Here's how the part is built. I have some questions about the finished solid (model axes, mm). Face numbers are marked on the shaded views. A direction names the side the tool comes from. Coordinates: 2 decimals unless noted, no trailing zeros. Loops run counter-clockwise (first coordinate to the right, second up) from the corner with the lowest first, then second, coordinate; pieces in that order, holes last. Notation, with made-up numbers: (29.25, 20.5) - (72.25, 20.5) arc R10 cw to (72.25, 24.5) - close; hole circle Ø7 at (18, 17). An arc over 180 degrees is marked (long way). Use a Markdown table: item, result.
```python
from build123d import *

# Parameters (mm, degrees)
SKETCH_W        = 59
SKETCH_H        = 60
PAD_DEPTH       = 11
SKETCH001_R     = 7.6
POCKET_DEPTH    = 60.001
SKETCH002_R     = 1.75
POCKET001_DEPTH = 11.001
POCKET002_DEPTH = 9
SKETCH004_R     = 2.25
POCKET003_DEPTH = 11.001
SKETCH008_R     = 4.1
POCKET005_DEPTH = 20
SKETCH010_W     = 20
SKETCH010_H     = 25
POCKET006_DEPTH = 5
SKETCH011_R     = 2.9
POCKET007_DEPTH = 3.5
CHAMFER_SIZE    = 3


with BuildPart() as part:
    # Sketch → Pad (new body)
    with BuildSketch(Plane.XY):
        with Locations((19.5, 0)):
            Rectangle(SKETCH_W, SKETCH_H)
    extrude(amount=PAD_DEPTH)

    # Sketch001 → Pocket (cut, through all)
    with BuildSketch(Plane.XZ.offset(30)):
        with Locations((0, 11)):
            Circle(SKETCH001_R)
    extrude(amount=-POCKET_DEPTH, mode=Mode.SUBTRACT)

    # Sketch002 → Pocket001 (cut, through all)
    with BuildSketch(Plane.XY.offset(11)):
        with Locations((-6, 27)):
            Circle(SKETCH002_R)
        with Locations((40, 27)):
            Circle(SKETCH002_R)
        with Locations((-6, -27)):
            Circle(SKETCH002_R)
        with Locations((40, -27)):
            Circle(SKETCH002_R)
        with Locations((6, 27)):
            Circle(SKETCH002_R)
        with Locations((6, -27)):
            Circle(SKETCH002_R)
        with Locations((6, 0)):
            Circle(SKETCH002_R)
        with Locations((-6, 0)):
            Circle(SKETCH002_R)
        with Locations((40, -13)):
            Circle(SKETCH002_R)
        with Locations((40, 13)):
            Circle(SKETCH002_R)
    extrude(amount=-POCKET001_DEPTH, mode=Mode.SUBTRACT)

    # Sketch003 → Pocket002 (cut)
    with BuildSketch(Plane.XY.offset(11)):
        with BuildLine():
            Line((10, 35), (10, -35))
            Line((10, -35), (32, -35))
            Line((32, -35), (32, -17.246794))
            ThreePointArc((32, -17.246794), (35.044647, -14.065445), (36.736695, -10))
            Line((36.736695, -10), (56.736695, -10))
            Line((56.736695, -10), (56.736695, 10))
            Line((56.736695, 10), (36.736695, 10))
            ThreePointArc((36.736695, 10), (35.044647, 14.065445), (32, 17.246794))
            Line((32, 17.246794), (32, 35))
            Line((32, 35), (10, 35))
        make_face()
    extrude(amount=-POCKET002_DEPTH, mode=Mode.SUBTRACT)

    # Sketch004 → Pocket003 (cut, through all)
    with BuildSketch(Plane(origin=(0, 0, 0), x_dir=(1, 0, 0), z_dir=(0, 0, -1))):
        with Locations((25, 7.5)):
            Circle(SKETCH004_R)
        with Locations((25, -7.5)):
            Circle(SKETCH004_R)
    extrude(amount=-POCKET003_DEPTH, mode=Mode.SUBTRACT)

    # Sketch008 → Pocket005 (cut)
    with BuildSketch(Plane.YZ.offset(49)):
        with Locations((-20, 11)):
            Circle(SKETCH008_R)
        with Locations((20, 11)):
            Circle(SKETCH008_R)
    extrude(amount=-POCKET005_DEPTH, mode=Mode.SUBTRACT)

    # Sketch010 → Pocket006 (cut)
    with BuildSketch(Plane.YZ.offset(49)):
        with Locations((0, 5.473744)):
            Rectangle(SKETCH010_W, SKETCH010_H)
    extrude(amount=-POCKET006_DEPTH, mode=Mode.SUBTRACT)

    # Sketch011 → Pocket007 (cut)
    with BuildSketch(Plane(origin=(0, 0, 0), x_dir=(1, 0, 0), z_dir=(0, 0, -1))):
        with Locations((6, 27)):
            Circle(SKETCH011_R)
        with Locations((40, -13)):
            Circle(SKETCH011_R)
        with Locations((-6, -27)):
            Circle(SKETCH011_R)
        with Locations((6, -27)):
            Circle(SKETCH011_R)
        with Locations((40, 27)):
            Circle(SKETCH011_R)
        with Locations((40, 13)):
            Circle(SKETCH011_R)
        with Locations((40, -27)):
            Circle(SKETCH011_R)
        with Locations((-6, 27)):
            Circle(SKETCH011_R)
        with Locations((6, 0)):
            Circle(SKETCH011_R)
        with Locations((-6, 0)):
            Circle(SKETCH011_R)
    extrude(amount=-POCKET007_DEPTH, mode=Mode.SUBTRACT)

    # Chamfer
    chamfer_edges = [part.edges().sort_by_distance(p)[0] for p in [
        (49, -10, 6.5),
        (49, 10, 6.5),
    ]]
    chamfer(chamfer_edges, length=CHAMFER_SIZE)


solid = part.part
```
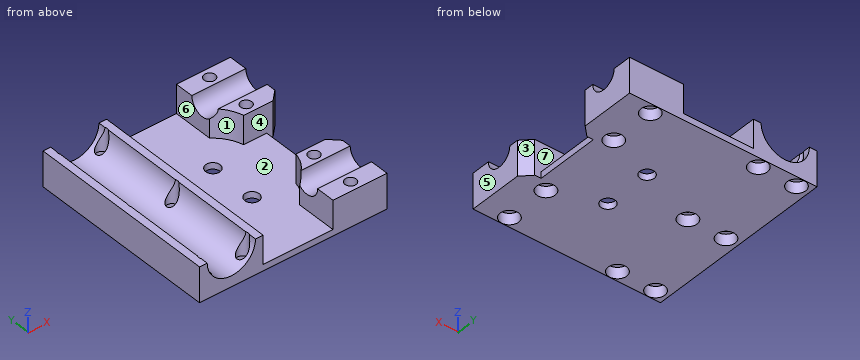
Q1. I want a section at B-B, the plane x = 5. Write out the boundary of the cut face in (y, z).
Check values:
| item | result |
|---|---|
| outline | (-30, 0) - (-29.72, 0) - (-29.72, 3.5) - (-28.44, 3.5) - (-28.44, 5.28) - (-30, 5.28) - close; (-25.56, 3.5) - (-24.28, 3.5) - (-24.28, 0) - (-2.72, 0) - (-2.72, 3.5) - (-1.44, 3.5) - (-1.44, 5.28) - (-25.56, 5.28) - close; (1.44, 3.5) - (2.72, 3.5) - (2.72, 0) - (24.28, 0) - (24.28, 3.5) - (25.56, 3.5) - (25.56, 5.28) - (1.44, 5.28) - close; (28.44, 3.5) - (29.72, 3.5) - (29.72, 0) - (30, 0) - (30, 5.28) - (28.44, 5.28) - close |
Q2. Which directions (+Z, -Z, +X, -X, +Y, -Y) give clear straight access to the entire face, cutting with the end or side of a thin tool? Please do the marked faces 5, 6 and 7.
Check values:
| item | result |
|---|---|
| face 5 | +Z, -Z, +X, +Y, -Y |
| face 6 | +Z, +Y, -Y |
| face 7 | +Z, +X |
Q3. I want a section at D-D, the plane x = 24. Write out the boundary of the cut face in (y, z), then the cut area to 3 significant figures.
Check values:
| item | result |
|---|---|
| outline | (-30, 0) - (-9.52, 0) - (-9.52, 2) - (-30, 2) - close; (-5.48, 0) - (5.48, 0) - (5.48, 2) - (-5.48, 2) - close; (9.52, 0) - (30, 0) - (30, 2) - (9.52, 2) - close |
| area | 104 mm^2 |
Q4. I want a section at A-A, the plane y = 7.5. Write out the boundary of the cut face in (x, z), then the cut area to 3 significant figures.
Check values:
| item | result |
|---|---|
| outline | (-10, 0) - (22.75, 0) - (22.75, 2) - (10, 2) - (10, 11) - (7.6, 11) arc R7.6 cw to (-7.6, 11) - (-10, 11) - close; (27.25, 0) - (44, 0) - (44, 2) - (27.25, 2) - close |
| area | 188 mm^2 |
Q5. Will these pins go through, and if not, where does the flat tip stop? P1, Ø4.5, axis at x = -6, y = 27, coming from the -Z side; P2, Ø10, axis at x = 29, y = 3.5, coming from the +Z side; P3, Ø3, axis at x = 6, y = 0, coming from the +Z side.
Check values:
| item | result |
|---|---|
| P1 | z = 3.5 |
| P2 | z = 2 |
| P3 | through |
Q6. I want a section at C-C, the plane y = -20. Write out the boundary of the cut face in (x, z), then the cut area to 3 significant figures.
Check values:
| item | result |
|---|---|
| outline | (-10, 0) - (49, 0) - (49, 6.9) - (32, 6.9) - (32, 2) - (10, 2) - (10, 11) - (7.6, 11) arc R7.6 cw to (-7.6, 11) - (-10, 11) - close |
| area | 291 mm^2 |
Q7. Please list where these lines run through material, in increasing order: L1, parallel to X at y = 0, z = 1; L2, parallel to X at y = 27, z = 1.15; L3, parallel to Y at x = 44, z = 2. Write a range as from..to.
Check values:
| item | result |
|---|---|
| L1 | -10..-8.9, -3.1..3.1, 8.9..44 |
| L2 | -10..-8.9, -3.1..3.1, 8.9..37.1, 42.9..49 |
| L3 | -30..-10, 10..30 |
Q8. If we mould it in two halves opening along X, with no side actions, what happens to the marked faces 1, 2, 3 and 4? For each: pulls with the +X half, pulls with the -X half, needs draft (parallel to the pull), parting line crosses it, or undercut.
Check values:
| item | result |
|---|---|
| face 1 | undercut |
| face 2 | undercut |
| face 3 | pulls with the +X half |
| face 4 | needs draft |
